Source: three-view drawing plus pictorial views. Frame: mm from the lowest corner of the part. A direction names the side the tool comes from. Coordinates: 2 decimals unless noted, no trailing zeros. Write each loop counter-clockwise with the first axis right and the second up, starting at its lowest first coordinate (ties: lowest second). Pieces come first, ordered by that corner, then holes. Notation, with made-up numbers: (-26, 64) - (17, 64) arc R22 ccw to (17, 100) - close; hole circle Ø7 at (44, 2.25). An arc over 180 degrees is marked (long way). One line per item, written item: value.
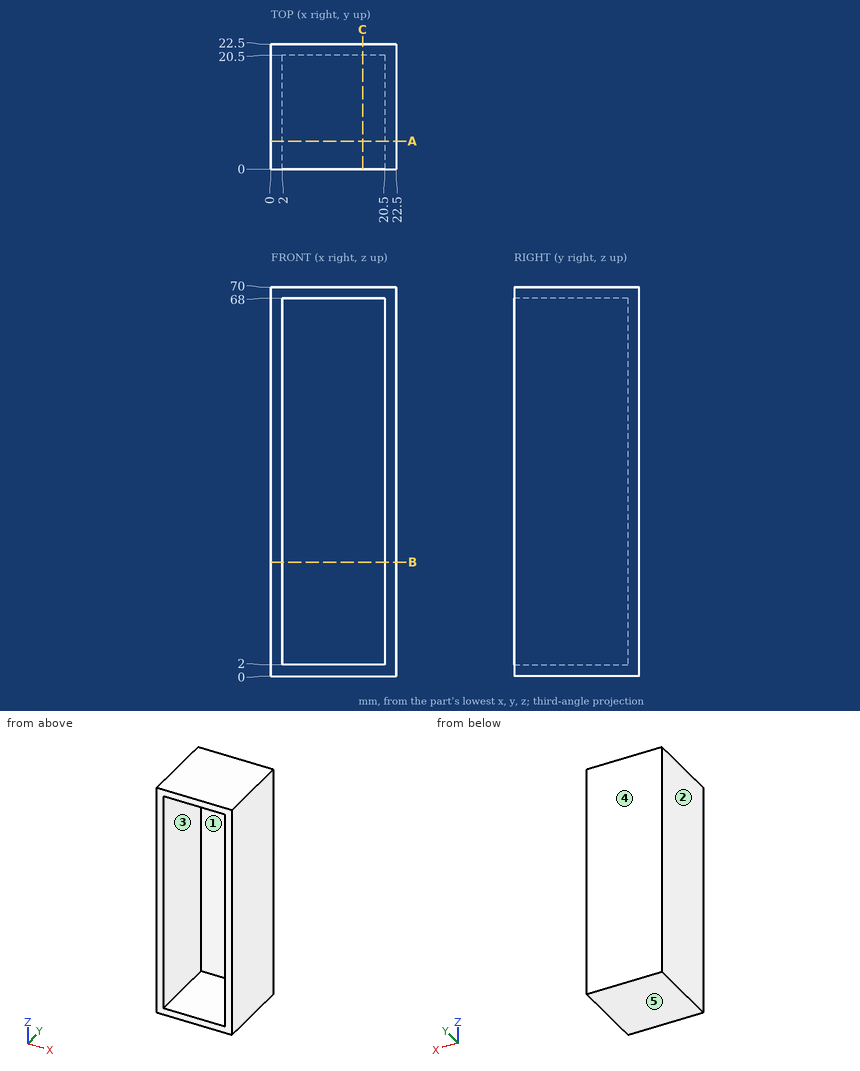
1) Reachability of the marked faces 1 and 2 from +Z, -Z, +X, -X, +Y, -Y: full face, straight path, thin tool, end or side. Return the list, or none.
Values found:
face 1: -Y
face 2: +Z, -Z, -X, +Y, -Y
2) Section query A-A on y = 5. Output: boundary loops of the cut face in (x, z).
Values found:
outline: (0, 0) - (22.5, 0) - (22.5, 70) - (0, 70) - close; hole (2, 2) - (20.5, 2) - (20.5, 68) - (2, 68) - close
3) Draft query along Z for the marked faces 3, 4 and 5. Return one class per face: released by +Z, released by -Z, zero draft, split by the parting line, or undercut.
Values found:
face 3: undercut
face 4: zero draft
face 5: released by -Z
4) Section query C-C on x = 16.5. Output: boundary loops of the cut face in (y, z), then the cut area to 3 significant figures.
Values found:
outline: (0, 0) - (22.5, 0) - (22.5, 70) - (0, 70) - (0, 68) - (20.5, 68) - (20.5, 2) - (0, 2) - close
area: 222 mm2
5) Material intervals for line 1 (Z direction, x = 17, y = 3.25); line 2 (X direction, y = 1, z = 31); line 3 (Y direction, x = 7.5, z = 3), sorted ascending.
Values found:
line 1: 0 to 2, 68 to 70
line 2: 0 to 2, 20.5 to 22.5
line 3: 20.5 to 22.5
6) Contact query for flat-ended pins moving along their axis: P1, Ø6, axis at y = 5.5, z = 37.5, coming from the -X side; P2, Ø9, axis at x = 7.5, z = 25, coming from the -Y side. Output: stop coordinate, or through.
Values found:
P1: x = 0
P2: y = 20.5
7) Section query B-B on z = 20.5. Output: boundary loops of the cut face in (x, y).
Values found:
outline: (0, 0) - (2, 0) - (2, 20.5) - (20.5, 20.5) - (20.5, 0) - (22.5, 0) - (22.5, 22.5) - (0, 22.5) - close
